Check sheet for the modelled part. Datum: model origin and axes. Units: mm. A direction names the side the tool comes from. Round coordinates to 2 decimals unless told otherwise and drop trailing zeros. Write each loop counter-clockwise with the first axis right and the second up, starting at its lowest first coordinate (ties: lowest second). Pieces come first, ordered by that corner, then holes. Notation, with made-up numbers: (83, 24.25) - (96, 24.25) arc R24 cw to (96, 60.25) - close; hole circle Ø3 at (44, 27.25). An arc over 180 degrees is marked (long way). Use one line per item in the form item = value. Start each with the question number.
1) Section check A-A (y = -40.5). Record the boundary of the cut face in (x, z) (3 decimals).
2) Gauge pin test, flat ends, axial feed: P1, Ø14, axis at y = 9, z = 8.5, coming from the +X side (3 decimals); P2, Ø4, axis at x = 14.5, y = -48, coming from the +Z side (3 decimals); P3, Ø11.5, axis at x = 50, z = 37.5, coming from the +Y side. Record the tip position at first contact, or that the pin passes through.
3) Scan lines: probe 1 along X at (y, z) = (33.5, 1) (3 decimals); probe 2 along Z at (x, y) = (-1, -55) (3 decimals); probe 3 along X at (y, z) = (24.5, 32) (3 decimals). Record each from-to range of solid material in increasing order.
4) Section check B-B (x = 78). Record the boundary of the cut face in (y, z), then the cut area to 3 significant figures.
5) Draft check along X on faces 1 (the face through (41.367, 1.763, 37.48)), 2 (the face through (22.225, 17, 23)), 3 (the face through (0, -63.5, 0)). Enter one of: +X half, -X half, draft (parallel to the pull), parting line (faces both ways), or undercut.
6) Set-up check for faces 4 (the face through (41.275, -1, 8)), 5 (the face through (34.93, -0.43, 61.21)), 6 (the face through (37, 25.4, 36)): record each of +Z, -Z, +X, -X, +Y, -Y from which the full face is reachable in a straight line by a thin tool's end or side.
from build123d import *

# Parameters (mm, degrees)
F1_DEPTH = 63.5
F2_DEPTH = 25.4
F3_DEPTH = 7.9375
F5_R     = 6.35


with BuildPart() as f1:
    # F0 (on Front) → F1 (new body, symmetric)
    with BuildSketch(Plane.XZ):
        Polygon((22.225, 9.525), (-41.275, 9.525), (-41.275, -9.525), (41.275, -9.525), (41.275, 9.525), align=None)
    extrude(amount=F1_DEPTH, both=True)

    # F0 (on Front) → F2 (join, symmetric)
    with BuildSketch(Plane.XZ):
        with BuildLine():
            Line((22.225, 36.372416), (22.225, 9.525))
            Line((22.225, 9.525), (41.275, 9.525))
            Line((41.275, 9.525), (41.275, 36.372416))
            ThreePointArc((41.275, 36.372416), (43.906682, 41.711138), (49.743862, 42.8752))
            Line((49.743862, 42.8752), (60.325, 42.8752))
            Line((60.325, 42.8752), (60.325, 61.9252))
            Line((60.325, 61.9252), (51.428748, 61.9252))
            add(Edge.make_bspline(
                [(39.172455, 60.59283), (43.120534, 61.049962), (47.205418, 61.485125), (51.428748, 61.9252)],
                knots=[97.106887, 97.106887, 97.106887, 97.106887, 106.488336, 106.488336, 106.488336, 106.488336], degree=3))
            ThreePointArc((39.172455, 60.59283), (26.882582, 51.152848), (22.225, 36.372416))
        make_face()
    extrude(amount=F2_DEPTH, both=True)

    # F0 (on Front) → F3 (join, symmetric)
    with BuildSketch(Plane.XZ):
        with BuildLine():
            add(Edge.make_bspline(
                [(-41.275, 9.525), (-27.90281, 48.775516), (-1.693912, 55.861078), (39.172455, 60.59283)],
                knots=[0, 0, 0, 0, 97.106887, 97.106887, 97.106887, 97.106887], degree=3))
            Line((-41.275, 9.525), (22.225, 9.525))
            Line((22.225, 9.525), (22.225, 36.372416))
            ThreePointArc((22.225, 36.372416), (26.882582, 51.152848), (39.172455, 60.59283))
        make_face()
    extrude(amount=F3_DEPTH, both=True)

    # F0 (on Front) → F4 (revolve)
    with BuildSketch(Plane.XZ):
        Polygon((85.725, 61.9252), (60.325, 61.9252), (60.325, 42.8752), (60.325, 38.1), (85.725, 38.1), align=None)
    revolve(axis=Axis((60.325, 0, 52.3875), (0, 0, -1)))

    # F5
    f5_edges = [f1.edges().sort_by_distance(p)[0] for p in [
        (41.275, -63.5, 0),
        (-41.275, -63.5, 0),
        (-41.275, 63.5, 0),
        (41.275, 63.5, 0),
    ]]
    fillet(f5_edges, radius=F5_R)


solid = f1.part
Results are:
q1.outline = (-41.275, -9.525) - (41.275, -9.525) - (41.275, 9.525) - (-41.275, 9.525) - close
q2.P1 = 41.275
q2.P2 = 9.525
q2.P3 = 25.4
q3.probe_1 = -41.275 to 41.275
q3.probe_2 = -9.525 to 9.525
q3.probe_3 = 22.225 to 41.275
q4.outline = (-18.24, 38.1) - (18.24, 38.1) - (18.24, 61.93) - (-18.24, 61.93) - close
q4.area = 869 mm²
q5.face_1 = undercut
q5.face_2 = -X half
q5.face_3 = draft
q6.face_4 = -Z, +X, +Y, -Y
q6.face_5 = +Z, -X
q6.face_6 = +Z, +X, -X, +Y
